from build123d import *

# Parameters (mm, degrees)
F0_R          = 38.1
F1_DEPTH      = 609.6
F2_R          = 9.525
F3_DEPTH      = 38.101
F3_DEPTH_BACK = 38.101
F4_R          = 15.875
F5_DEPTH      = 609.6010001


with BuildPart() as f1:
    # F0 (on Front) → F1 (new body)
    with BuildSketch(Plane.XZ):
        Circle(F0_R)
    extrude(amount=F1_DEPTH)

    # F2 (on Right) → F3 (cut, two sides)
    with BuildSketch(Plane.YZ) as f3_sk:
        with Locations((-25.4, 0)):
            Circle(F2_R)
    extrude(amount=-F3_DEPTH, mode=Mode.SUBTRACT)
    extrude(f3_sk.sketch, amount=F3_DEPTH_BACK, mode=Mode.SUBTRACT)

    # F4 (on Front) → F5 (cut, through all)
    with BuildSketch(Plane.XZ):
        Circle(F4_R)
    extrude(amount=F5_DEPTH, mode=Mode.SUBTRACT)


solid = f1.part
The model under review builds one solid part; all positions refer to its coordinate system, in mm. Round coordinates to 2 decimals unless told otherwise and drop trailing zeros. Loops run counter-clockwise (first coordinate to the right, second up) from the corner with the lowest first, then second, coordinate; pieces in that order, holes last. Notation, with made-up numbers: (31, 41.5) - (75, 41.5) arc R24 cw to (75, 65.5) - close; hole circle Ø6 at (3.25, 75.25). An arc over 180 degrees is marked (long way). Use CSV: the item, a comma, the result in double quotes.
(1) Take a section at B-B, the plane x = 0. Give the boundary of the cut face in (y, z) (3 decimals).
Working result:
outline,"(-609.6, -38.1) - (0, -38.1) - (0, -15.875) - (-609.6, -15.875) - close; (-609.6, 15.875) - (0, 15.875) - (0, 38.1) - (-609.6, 38.1) - close"
(2) Take a section at A-A, the plane z = 0. Give the boundary of the cut face in (x, y) (3 decimals), plus the area to 4 significant figures.
Working result:
outline,"(-38.1, -609.6) - (-15.875, -609.6) - (-15.875, -34.925) - (-38.1, -34.925) - close; (-38.1, -15.875) - (-15.875, -15.875) - (-15.875, 0) - (-38.1, 0) - close; (15.875, -609.6) - (38.1, -609.6) - (38.1, -34.925) - (15.875, -34.925) - close; (15.875, -15.875) - (38.1, -15.875) - (38.1, 0) - (15.875, 0) - close"
area,"26,250 mm^2"
(3) Take a section at D-D, the plane z = -31.5. Give the boundary of the cut face in (x, y), plus the area to 3 significant figures.
Working result:
outline,"(-21.43, -609.6) - (21.43, -609.6) - (21.43, 0) - (-21.43, 0) - close"
area,"26,100 mm^2"
(4) Clearance check with flat-ended pins moving along their axes: P1, Ø1.5, axis at x = -17.5, y = -153, coming from the -Z side; P2, Ø15, axis at y = -25.4, z = 0, coming from the +X side; P3, Ø2, axis at y = -352.5, z = 17.5, coming from the +X side; P4, Ø4, axis at y = -519.5, z = -18, coming from the -X side. State where each tip first meets the part, or that it passes through.
Working result:
P1,"stops at z = -34.22"
P2,"passes through"
P3,"stops at x = 34.34"
P4,"stops at x = -34.58"
(5) Take a section at C-C, the plane y = -51.5. Give the boundary of the cut face in (x, z) (3 decimals).
Working result:
outline,"circle Ø76.2 at (0, 0); hole circle Ø31.75 at (0, 0)"
(6) The part is to be moulded in two halves that separate along Z. For faces 1 (the flat face through (16, -609.6, 1)), 2 (the cylindrical face through (36.34, -300.53, 11.44)), 3 (the cylindrical face through (-15.86, -300.53, 0.7)), 4 (the cylindrical face through (25.22, -16.6, -3.65)), say which applies: pulls with the +Z half, pulls with the -Z half, needs draft (parallel to the pull), parting line crosses it, or undercut.
Working result:
face 1,"needs draft"
face 2,"parting line crosses it"
face 3,"undercut"
face 4,"undercut"
(7) For line 1 (Z direction, x = -1, y = -38); line 2 (X direction, y = -208, z = 0) (3 decimals), list the stretches that pass through material, from the lowest coordinate up.
Working result:
line 1,"z = -38.09 to -15.84, 15.84 to 38.09"
line 2,"x = -38.1 to -15.875, 15.875 to 38.1"
